Autodesk Inventor part; units mm, degrees
ref_plane "YZ Plane" through (0, 0, 0) normal (1, 0, 0) x (0, 1, 0)
ref_plane "XZ Plane" through (0, 0, 0) normal (0, 1, 0) x (-1, 0, 0)
ref_plane "XY Plane" through (0, 0, 0) normal (0, 0, 1) x (1, 0, 0)
sketch "Sketch1" plane through (0, 0, 0) normal (0, 1, 0) x (-1, 0, 0)
  line L0 (0, 25) -> (0, -25) construction
  line L1 (-3.5, 25) -> (-3.5, -25)
  line L2 (3.5, -25) -> (3.5, 25)
  arc A0 (3.5, 25) -> (-3.5, 25) centre (0, 25) ccw
  arc A1 (-3.5, -25) -> (3.5, -25) centre (0, -25) ccw
  point P0 (0, 0)
  point P1 (0, 0)
  dimension "d0" = 50
  dimension "d1" = 7
extrude "Extrusion1" add sketch "Sketch1" along normal blind 3.75
sketch "Sketch2" plane through (0, 3.75, 0) normal (0, 1, 0) x (1, 0, 0)
  arc A0 (3.5, 25) -> (-3.5, 25) centre (0, 25) ccw
  line L0 (-3.5, 25) -> (-3.5, -25)
  arc A1 (-3.5, -25) -> (3.5, -25) centre (0, -25) ccw
  line L1 (3.5, -25) -> (3.5, 25)
  circle A2 centre (0, 25) radius 1.5
  circle A3 centre (0, -25) radius 1.5
  arc A4 (-3.5, -25) -> (3.5, -25) centre (0, -25) ccw
  point P0 (0, 0)
  dimension "d38" = 3
  dimension "d39" = 3
sketch "Sketch3" plane through (0, 0, 0) normal (0, -1, 0) x (1, 0, 0)
  arc A0 (-3.5, -25) -> (3.5, -25) centre (0, -25) ccw
  line L0 (3.5, 25) -> (3.5, -25)
  arc A1 (3.5, 25) -> (-3.5, 25) centre (0, 25) ccw
  line L1 (-3.5, -25) -> (-3.5, 25)
  circle A2 centre (0, 0) radius 2.5
  circle A3 centre (0, 0) radius 1.2
  dimension "d11" = 5
  dimension "d14" = 2.4
extrude "Extrusion2" add sketch "Sketch3" along normal blind 7 contours A2 | A3
sketch "Sketch5" plane through (0, -7, 0) normal (0, -1, 0) x (1, 0, 0)
  point P0 (0, 0)
  point P1 (0, 0)
hole "Hole2" at (0, -7, 0) direction (0, 1, 0) diameter 2.4 depth 10 tip angle 118
sketch "Sketch6" plane through (0, 3.75, 0) normal (0, 1, 0) x (1, 0, 0)
  point P0 (0, 0)
  point P1 (0, 0)
hole "Hole3" at (0, 3.75, 0) direction (0, -1, 0) diameter 5.2 depth 1.5
sketch "Sketch8" plane through (0, 0, 0) normal (0, -1, 0) x (1, 0, 0)
  circle A0 centre (0, 0) radius 2.5
  arc A1 (-3.5, -25) -> (3.5, -25) centre (0, -25) ccw
  line L0 (3.5, 25) -> (3.5, -25)
  arc A2 (3.5, 25) -> (-3.5, 25) centre (0, 25) ccw
  line L1 (-3.5, -25) -> (-3.5, 25)
  line L2 (3.5, 25) -> (3.5, -25)
  line L3 (3.5, -13.5) -> (3.5, -16) construction
  line L4 (0.75, -13.5) -> (0.75, -16)
  line L5 (6.25, -16) -> (6.25, -13.5)
  arc A3 (6.25, -13.5) -> (0.75, -13.5) centre (3.5, -13.5) ccw
  arc A4 (0.75, -16) -> (6.25, -16) centre (3.5, -16) ccw
  line L6 (-5.2, 0) -> (6.7, 0)
  line L7 (3.5, 13.5) -> (3.5, 16) construction
  line L8 (0.75, 13.5) -> (0.75, 16)
  line L9 (6.25, 16) -> (6.25, 13.5)
  arc A5 (0.75, 13.5) -> (6.25, 13.5) centre (3.5, 13.5) ccw
  arc A6 (6.25, 16) -> (0.75, 16) centre (3.5, 16) ccw
  point P0 (3.5, -14.75)
  point P1 (3.5, -18.75)
  point P2 (3.5, -10.75)
  point P3 (3.5, 14.75)
  point P4 (3.5, 10.75)
  point P5 (3.5, 18.75)
  dimension "d32" = 2.5
  dimension "d33" = 5.5
  dimension "d71" = 13.5
extrude "Cut" cut sketch "Sketch8" against normal through all contours A5 L8 A6 L0 | L0 A4 L4 A3
fillet "Fillet1" radius 2 4 edges at (3.5, 1.875, -10.75) (3.5, 1.875, -18.75) (3.5, 1.875, 18.75) (3.5, 1.875, 10.75)
extrude "Extrusion5" [suppressed]
sketch "Sketch9" plane through (0, 9.55, -25) normal (0, 1, 0) x (1, 0, 0)
  circle A0 centre (0, 0) radius 1.5
  circle A1 centre (0, -50) radius 1.5
  circle A2 centre (0, -50) radius 1.5
  circle A3 centre (0, -50) radius 1.85
  circle A4 centre (0, 0) radius 1.5
  circle A5 centre (0, 0) radius 1.85
  point P0 (0, -25)
  dimension "d42" = 3.7
  dimension "d43" = 3.7
extrude "Extrusion6" [suppressed]
chamfer "Chamfer1" [suppressed]
fillet "Fillet2" [suppressed]
sketch "Sketch10" plane through (0, 0, 0) normal (0, -1, 0) x (1, 0, 0)
  arc A0 (3.5, 25) -> (-3.5, 25) centre (0, 25) ccw
  arc A1 (-3.5, -25) -> (3.5, -25) centre (0, -25) ccw
  circle A2 centre (0, 25) radius 2.25
  circle A3 centre (0, -25) radius 2.25
  point P0 (0, 0)
  dimension "d50" = 4.5
extrude "Extrusion7" add sketch "Sketch10" along normal blind 4
sketch "Sketch11" plane through (0, -4, 25) normal (0, -1, 0) x (1, 0, 0)
  circle A0 centre (0, 0) radius 2.25
  circle A1 centre (0, -50) radius 2.25
  circle A2 centre (0, 0) radius 2.4
  circle A3 centre (0, -50) radius 2.4
  point P0 (0, -25)
  dimension "d54" = 4.8
  dimension "d70" = 4.5
extrude "Extrusion8" add sketch "Sketch11" along normal blind 0.4 contours A0 | A1 | A2 | A3
fillet "Fillet3" radius 0.4 2 edges at (-2.25, -4, 25) (-2.25, -4, -25)
fillet "Fillet4" radius 0.8 3 edges at (-2.25, 0, 25) (-2.25, 0, -25) (-2.5, 0, 0)
sketch "Sketch13" plane through (0, 3.75, 0) normal (0, 1, 0) x (1, 0, 0)
  circle A0 centre (0, -25) radius 2.4
  circle A1 centre (0, 25) radius 2.25
  circle A2 centre (0, -25) radius 3.05
  point P0 (0, 0)
hole "Hole4" at (0, 3.75, 25) at (0, 3.75, -25) direction (0, -1, 0) diameter 2.2 end through all counterbore diameter 3.6 counterbore depth 1.5
equation "\"d43\" = d42"
properties part number "ActuatorLink"
The model under review builds one solid part; all positions refer to its coordinate system, in mm. A direction names the side the tool comes from. Round coordinates to 2 decimals unless told otherwise and drop trailing zeros. Loops run counter-clockwise (first coordinate to the right, second up) from the corner with the lowest first, then second, coordinate; pieces in that order, holes last. Notation, with made-up numbers: (33, 82.5) -> (65, 82.5) arc R28 ccw to (65, 110.5) -> close; hole circle Ø5 at (14.5, -11). An arc over 180 degrees is marked (long way). One line per question, with ' | ' between items. Start each with the question number.
Item 1: Wall thickness on line 1 along Z through (x, y) = (0, -4); line 2 along Z through (x, y) = (0, 3.1); line 3 along Z through (x, y) = (-0.5, -1.75): over which ranges is each line inside the solid? List them lowest first. Write a range as [from, to].
Item 2: Add section C-C, the plane x = 0. Count the separate pieces of the cut face and the enclosed holes in it, then the cut area to 3 significant figures.
Item 3: For pin 1 (5 mm diameter, centred on y = -5, z = -2, fed in from -X); pin 2 (2 mm diameter, centred on y = 2.5, z = 14.5, fed in from +X); pin 3 (3 mm diameter, centred on x = 0, z = 25, fed in from -Y); pin 4 (1.5 mm diameter, centred on y = -0.5, z = -18.5, fed in from -X), all flat-tipped, find the tip position at first contact; note any pin that passes through.
Item 4: Add section A-A, the plane y = 1. Write out the cut boundary in (x, z), then the cut area to 3 significant figures.
Item 5: Machinability: for faces 1 (the face through (0.75, 2, 15)), 2 (the face through (-0.52, -4.197, 27.343)), 3 (the face through (-0.488, -2.224, 27.196)), 4 (the face through (1, 2.25, 1)), which of the approach directions +Z, -Z, +X, -X, +Y, -Y give a long, thin tool a straight path to every point of the face, cutting with its end or side? Answer none if there is none.
Item 6: Add section D-D, the plane z = -15. Write out the cut boundary in (x, y), then the cut area to 3 significant figures.
Item 7: Add section B-B, the plane z = 0. Write out the cut boundary in (x, y), then the cut area to 3 significant figures.
Item 8: Draft analysis for pull direction X (two halves, no side actions). For faces 5 (the face through (-0.541, 2.99, 26.717)), 6 (the face through (3.18, 1.9, 10.28)), 7 (the face through (-0.52, -4.197, -22.657)), state which applies: +X half, -X half, draft (parallel to the pull), parting line (faces both ways), or undercut.
Return value:
1) line 1: z = [-27.4, -26.1], [-23.9, -22.6], [-2.5, -1.2], [1.2, 2.5], [22.6, 23.9], [26.1, 27.4] | line 2: z = [-28.5, -26.8], [-23.2, -2.6], [2.6, 23.2], [26.8, 28.5] | line 3: z = [-27.19, -25.98], [-24.02, -22.81], [-2.45, -1.09], [1.09, 2.45], [22.81, 24.02], [25.98, 27.19]
2) separate pieces: 4 | enclosed holes: 0 | area: 219 mm2
3) pin 1: stops at x = -2.5 | pin 2: stops at x = 0.75 | pin 3: stops at y = -4.4 | pin 4: stops at x = -3.5
4) outline: (-3.5, -25) arc R3.5 ccw to (3.5, -25) -> (3.5, -20.31) arc R2 ccw to (2.34, -18.49) arc R2.75 cw to (0.75, -16) -> (0.75, -13.5) arc R2.75 cw to (2.34, -11.01) arc R2 ccw to (3.5, -9.19) -> (3.5, 9.19) arc R2 ccw to (2.34, 11.01) arc R2.75 cw to (0.75, 13.5) -> (0.75, 16) arc R2.75 cw to (2.34, 18.49) arc R2 ccw to (3.5, 20.31) -> (3.5, 25) arc R3.5 ccw to (-3.5, 25) -> close; hole circle Ø2.4 at (0, 0); hole circle Ø2.2 at (0, -25); hole circle Ø2.2 at (0, 25) | area: 337 mm2
5) face 1: +X, +Y, -Y | face 2: -Y | face 3: none | face 4: +Y
6) outline: (-3.5, 0) -> (0.75, 0) -> (0.75, 3.75) -> (-3.5, 3.75) -> close | area: 15.9 mm2
7) outline: (-3.5, 0) -> (-3.3, 0) arc R0.8 cw to (-2.5, -0.8) -> (-2.5, -7) -> (-1.2, -7) -> (-1.2, 2.25) -> (-2.6, 2.25) -> (-2.6, 3.75) -> (-3.5, 3.75) -> close; (1.2, -7) -> (2.5, -7) -> (2.5, -0.8) arc R0.8 cw to (3.3, 0) -> (3.5, 0) -> (3.5, 3.75) -> (2.6, 3.75) -> (2.6, 2.25) -> (1.2, 2.25) -> close | area: 31.5 mm2
8) face 5: undercut | face 6: +X half | face 7: parting line
